Input: part model. Units: mm. Frame: model coordinates. A direction names the side the tool comes from. Coordinates: 2 decimals unless noted, no trailing zeros. Order: outer loops, then holes, each group sorted by start corner. A loop starts at its lowest first (then second) coordinate and runs counter-clockwise, first axis right, second up.
from build123d import *

# Parameters (mm, degrees)
BOSS_EXTRUDE1_DEPTH = 70
FILLET1_R           = 1
FILLET2_R           = 1
FILLET3_R           = 1
FILLET4_R           = 1
FILLET5_R           = 1


with BuildPart() as part:
    # Sketch1 → Boss-Extrude1 (new body)
    with BuildSketch(Plane.XY):
        with BuildLine():
            Line((-30, 0), (-35, 0))
            ThreePointArc((-35, 0), (-24.366509464, -25.125151075), (1.07275523, -34.983556083))
            Line((1.07275523, -34.983556083), (1.913239039, -40.440769755))
            Line((1.913239039, -40.440769755), (-40.664590355, -40.440769755))
            Line((-40.664590355, -40.440769755), (-41.611505919, -45.440769755))
            Line((-41.611505919, -45.440769755), (9.356298233, -45.440769755))
            Line((9.356298233, -45.440769755), (6.644574503, -34.363492687))
            Line((6.644574503, -34.363492687), (5.454004631, -29.500064974))
            ThreePointArc((5.454004631, -29.500064974), (-2.399349656, -29.903898094), (-10.087846616, -28.253059138))
            ThreePointArc((-10.087846616, -28.253059138), (-12.915959233, -29.413373854), (-13.975418711, -26.545953964))
            ThreePointArc((-13.975418711, -26.545953964), (-14.748247142, -26.124494373), (-15.508377464, -25.680541825))
            ThreePointArc((-15.508377464, -25.680541825), (-18.510827542, -26.254862942), (-18.978488477, -23.233961675))
            ThreePointArc((-18.978488477, -23.233961675), (-19.65199094, -22.66714036), (-20.308573214, -22.080802839))
            ThreePointArc((-20.308573214, -22.080802839), (-23.365262749, -22.046157513), (-23.222418703, -18.99261092))
            ThreePointArc((-23.222418703, -18.99261092), (-23.7696551, -18.303100733), (-24.296426035, -17.59783174))
            ThreePointArc((-24.296426035, -17.59783174), (-27.285087446, -16.955605782), (-26.537452182, -13.991555728))
            ThreePointArc((-26.537452182, -13.991555728), (-26.936533055, -13.206937077), (-27.312421814, -12.410947371))
            ThreePointArc((-27.312421814, -12.410947371), (-30.113508646, -11.186829821), (-28.790987573, -8.430838306))
            ThreePointArc((-28.790987573, -8.430838306), (-29.025949689, -7.582495937), (-29.235920721, -6.727625107))
            ThreePointArc((-29.235920721, -6.727625107), (-31.737389499, -4.970580666), (-29.892883462, -2.532887353))
            ThreePointArc((-29.892883462, -2.532887353), (-29.973208903, -1.267575668), (-30, 0))
        make_face()
    extrude(amount=-BOSS_EXTRUDE1_DEPTH)

    # Fillet1
    fillet1_edges = [part.edges().sort_by_distance(p)[0] for p in [
        (5.454004631, -29.500064974, -35),
        (9.356298233, -45.440769755, -35),
        (-41.611505919, -45.440769755, -35),
        (-40.664590355, -40.440769755, -35),
        (1.913239039, -40.440769755, -35),
        (1.07275523, -34.983556083, -35),
        (-35, 0, -35),
    ]]
    fillet(fillet1_edges, radius=FILLET1_R)

    # Fillet2
    fillet2_edges = [part.edges().sort_by_distance(p)[0] for p in [
        (-29.892883462, -2.532887353, -35),
        (-28.790987573, -8.430838306, -35),
        (-26.537452182, -13.991555728, -35),
        (-23.222418703, -18.99261092, -35),
        (-18.978488477, -23.233961675, -35),
        (-13.975418711, -26.545953964, -35),
    ]]
    fillet(fillet2_edges, radius=FILLET2_R)

    # Fillet3
    fillet3_edges = [part.edges().sort_by_distance(p)[0] for p in [
        (-20.308573214, -22.080802839, -35),
        (-15.508377464, -25.680541825, -35),
        (-10.087846616, -28.253059138, -35),
    ]]
    fillet(fillet3_edges, radius=FILLET3_R)

    # Fillet4
    fillet4_edges = [part.edges().sort_by_distance(p)[0] for p in [
        (-27.312421814, -12.410947371, -35),
        (-24.296426035, -17.59783174, -35),
    ]]
    fillet(fillet4_edges, radius=FILLET4_R)

    # Fillet5
    fillet5_edges = [part.edges().sort_by_distance(p)[0] for p in [
        (-29.235920721, -6.727625107, -35),
    ]]
    fillet(fillet5_edges, radius=FILLET5_R)


solid = part.part
Item 1: Cut plane A-A on x = -11.5. Return loops of the section in (y, z), then the cut area to 3 significant figures.
Response values:
outline: (-45.44, -70) - (-40.44, -70) - (-40.44, 0) - (-45.44, 0) - close; (-33.06, -70) - (-29.52, -70) - (-29.52, 0) - (-33.06, 0) - close
area: 598 mm2
Item 2: Cut plane C-C on x = -18. Return loops of the section in (y, z), then the cut area to 3 significant figures.
Response values:
outline: (-45.44, -70) - (-40.44, -70) - (-40.44, 0) - (-45.44, 0) - close; (-30.02, -70) - (-26.52, -70) - (-26.52, 0) - (-30.02, 0) - close
area: 595 mm2
Item 3: Draft query along Y for faces 1 (the face through (-27.264, -16.988, -34.51)), 2 (the face through (-13, -31, -70)), 3 (the face through (-2.364, -29.907, -34.51)). Return one class per face: pulls with the +Y half, pulls with the -Y half, needs draft (parallel to the pull), parting line crosses it, or undercut.
Response values:
face 1: undercut
face 2: needs draft
face 3: pulls with the +Y half
Item 4: Pin query (flat end, axial travel): pin 1 Ø12 at (x, y) = (-34, -32.5) entering from -Z; pin 2 Ø1 at (y, z) = (-26.5, -54) entering from +X; pin 3 Ø6 at (y, z) = (-21, -20) entering from -X. Return the tip coordinate at first contact, or that it passes through.
Response values:
pin 1: passes through
pin 2: stops at x = -14.16
pin 3: stops at x = -30.02
Item 5: Ray query, probe 1 along Y at (x, z) = (-32, -55.5); probe 2 along Y at (x, z) = (-6.5, -5); probe 3 along X at (y, z) = (-9.5, -50.5). Return the intervals inside material, ascending.
Response values:
probe 1: y = -45.44 to -40.44, -14.18 to 0
probe 2: y = -45.44 to -40.44, -34.39 to -29.29
probe 3: x = -33.69 to -30.02
Item 6: Cut plane B-B on y = -21.5. Return loops of the section in (x, z).
Response values:
outline: (-27.62, -70) - (-23.74, -70) - (-23.74, 0) - (-27.62, 0) - close
Item 7: Access query for faces 4 (the face through (1.467, -37.544, -34.51)), 5 (the face through (-13, -31, 0)). Directions: +Z, -Z, +X, -X, +Y, -Y. A direction counts if a zero-diameter tool reaches every point of the face in a straight line with its end or side. Return the directions, or none.
Response values:
face 4: +Z, -Z, -X
face 5: +Z, +X, -X, +Y, -Y
